```python
from build123d import *

# Parameters (mm, degrees)
SKETCH1_R             = 16.916621232
BOSS_EXTRUDE1_DEPTH   = 64
SKETCH2_W             = 106.262974488
SKETCH2_H             = 38.987679284
BOSS_EXTRUDE2_DEPTH   = 10
BODY_MOVE_COPY1_ANGLE = 47


with BuildPart() as part:
    # Sketch1 → Boss-Extrude1 (new body)
    with BuildSketch(Plane(origin=(0, 0, 0), x_dir=(1, 0, 0), z_dir=(0, 1, 0))):
        with Locations((22.72979363, -8.239550191)):
            Circle(SKETCH1_R)
    extrude(amount=BOSS_EXTRUDE1_DEPTH)

    # Sketch2 → Boss-Extrude2 (add)
    with BuildSketch(Plane(origin=(0, 64, 0), x_dir=(1, 0, 0), z_dir=(0, 1, 0))):
        with Locations((22.72979363, -8.239550191)):
            Rectangle(SKETCH2_W, SKETCH2_H)
    extrude(amount=BOSS_EXTRUDE2_DEPTH)


with BuildPart() as part_1:
    # Body-Move/Copy1: moved
    add(part.part.rotate(Axis((22.72979363, 0, 8.239550191), (0, 1, 0)), BODY_MOVE_COPY1_ANGLE))


solid = part_1.part
```
Read the model definition and answer for the solid it produces. Units are mm, in the model's axes. A direction names the side the tool comes from. Give positions to 0.01 mm unless a question says otherwise; leave off trailing zeros. Order: outer loops, then holes, each group sorted by start corner. A loop starts at its lowest first (then second) coordinate and runs counter-clockwise, first axis right, second up.
(1) For faces 1 (the flat face through (59.2, 68.9, -30.4)), 2 (the flat face through (9, 64, -3)), determine the directions among +Z, -Z, +X, -X, +Y, -Y from which every point of the face is accessible in a straight line to the end or side of a thin tool.
(2) Find section B-B (z = 38). Give the vertices of the cut face in (x, y).
(3) Find section D-D (x = 27). Give the vertices of the cut face in (y, z), plus the area to 3 significant figures.
(4) Given pin 1 (12 mm diameter, centred on x = 4, z = 35.5, fed in from -Y); pin 2 (1.5 mm diameter, centred on y = 11, z = 14, fed in from +X); pin 3 (2 mm diameter, centred on y = 62, z = 12.5, fed in from +X), each flat-ended and moving along its own axis, determine where each tip first touches the part or whether it passes through.
(5) Find section C-C (y = 21). Give the vertices of the cut face in (x, z).
(6) Find section A-A (x = 14.5). Give the vertices of the cut face in (y, z).
(7) Straight lines are drawn through the part: L1, parallel to Y at x = 6, z = 40; L2, parallel to X at y = 69, z = -30; L3, parallel to Z at x = 33, y = 40.5. For each, find the intervals that lie inside material, in ascending order.
Result sheet:
1. face 1: -Z, +X, +Y, -Y
1. face 2: -Y
2. outline: (-23.26, 64) - (21.63, 64) - (21.63, 74) - (-23.26, 74) - close
3. outline: (0, -8.13) - (64, -8.13) - (64, -24.92) - (74, -24.92) - (74, 32.24) - (64, 32.24) - (64, 24.61) - (0, 24.61) - close
3. area: 2,670 mm2
4. pin 1: stops at y = 64
4. pin 2: stops at x = 38.89
4. pin 3: stops at x = 39.33
5. outline: circle Ø33.83 at (22.73, 8.24)
6. outline: (0, -6.54) - (64, -6.54) - (64, -11.52) - (74, -11.52) - (74, 45.65) - (64, 45.65) - (64, 23.02) - (0, 23.02) - close
7. L1: y = 64 to 74
7. L2: x = 31.73 to 59.63
7. L3: z = -5.2 to 21.68
